```python
from build123d import *

# Parameters (mm, degrees)
SKETCH1_W                        = 144
SKETCH1_H                        = 64
BOSS_EXTRUDE1_DEPTH              = 16
SKETCH3_W                        = 26
SKETCH3_H                        = 64
BOSS_EXTRUDE2_DEPTH              = 36
CHAMFER1_SIZE                    = 16
CUT_EXTRUDE1_REACH               = 146
SKETCH5_R                        = 8
BOSS_EXTRUDE3_DEPTH              = 22
FILLET1_R                        = 3
TAP_DRILL_FOR_M6_HELICOIL2_D     = 6.25
TAP_DRILL_FOR_M6_HELICOIL2_DEPTH = 10
TAP_DRILL_FOR_M6_HELICOIL2_TIP   = 1.877689434


with BuildPart() as part:
    # Sketch1 → Boss-Extrude1 (new body)
    with BuildSketch(Plane(origin=(0, 0, 0), x_dir=(1, 0, 0), z_dir=(0, 1, 0))):
        Rectangle(SKETCH1_W, SKETCH1_H)
    extrude(amount=BOSS_EXTRUDE1_DEPTH)

    # Sketch3 → Boss-Extrude2 (add)
    with BuildSketch(Plane(origin=(0, 16, 0), x_dir=(1, 0, 0), z_dir=(0, 1, 0))):
        with Locations((-59, 0)):
            Rectangle(SKETCH3_W, SKETCH3_H)
    extrude(amount=BOSS_EXTRUDE2_DEPTH)

    # Chamfer1
    chamfer1_edges = [part.edges().sort_by_distance(p)[0] for p in [
        (-72, 52, 0),
    ]]
    chamfer(chamfer1_edges, length=CHAMFER1_SIZE)

    # Sketch2 → Cut-Extrude1 (cut, up to next)
    with BuildSketch(Plane(origin=(72, 0, 0), x_dir=(0, 0, -1), z_dir=(1, 0, 0)), mode=Mode.PRIVATE) as cut_extrude1_sk1:
        Polygon((-16, 0), (-16, 7), (-8, 7), (-8, 16), (8, 16), (8, 7), (16, 7), (16, 0), align=None)
    cut_extrude1_tool1 = extrude(cut_extrude1_sk1.sketch, amount=-CUT_EXTRUDE1_REACH, mode=Mode.PRIVATE) & part.part
    add(cut_extrude1_tool1.solids().sort_by_distance((72, 6.630435, 0))[0], mode=Mode.SUBTRACT)

    # Sketch5 → Boss-Extrude3 (add)
    with BuildSketch(Plane(origin=(72, 0, 0), x_dir=(0, 0, -1), z_dir=(1, 0, 0))):
        with BuildLine():
            Line((-14.413228488, 42.946858611), (-27.401020705, 16))
            Line((-27.401020705, 16), (26.567243493, 16))
            Line((26.567243493, 16), (14.586247124, 42.575818949))
            ThreePointArc((14.586247124, 42.575818949), (0.204698485, 51.998690525), (-14.413228488, 42.946858611))
        make_face()
        with Locations((0, 36)):
            Circle(SKETCH5_R, mode=Mode.SUBTRACT)
    extrude(amount=-BOSS_EXTRUDE3_DEPTH)

    # Fillet1
    fillet1_edges = [part.edges().sort_by_distance(p)[0] for p in [
        (61, 16, -26.567243493),
        (61, 16, 27.401020705),
    ]]
    fillet(fillet1_edges, radius=FILLET1_R)

    # Tap Drill for M6 Helicoil2
    with Locations(Plane(origin=(-36, 0, 22), x_dir=(0, 0, -1), z_dir=(0, -1, 0))):
        with Locations((0, 0), (0, 70), (44, 0), (44, 70)):
            Hole(TAP_DRILL_FOR_M6_HELICOIL2_D / 2, depth=TAP_DRILL_FOR_M6_HELICOIL2_DEPTH)
            with Locations((0, 0, -(TAP_DRILL_FOR_M6_HELICOIL2_DEPTH + TAP_DRILL_FOR_M6_HELICOIL2_TIP / 2))):  # 118° drill point
                Cone(0, TAP_DRILL_FOR_M6_HELICOIL2_D / 2, TAP_DRILL_FOR_M6_HELICOIL2_TIP, mode=Mode.SUBTRACT)


solid = part.part
```
Part model, mm, in its own coordinate system. A direction names the side the tool comes from. Round coordinates to 2 decimals unless told otherwise and drop trailing zeros. Write each loop counter-clockwise with the first axis right and the second up, starting at its lowest first coordinate (ties: lowest second). Pieces come first, ordered by that corner, then holes. Notation, with made-up numbers: (83.5, 8.25) -> (119.5, 8.25) arc R20 ccw to (119.5, 16.25) -> close; hole circle Ø1 at (41.5, 58.5). An arc over 180 degrees is marked (long way). Return JSON: item names as keys, results as strings. Group by question number.
Q1. Probe L1, parallel to X at y = 3.75, z = 22 (3 decimals); L2, parallel to Z at x = 34, y = 5 (3 decimals); L3, parallel to Z at x = 65, y = 14. List the from-to ranges inside material, lowest first. Write a range as [from, to].
Q2. Mould opens along X. For faces 5 (the flat face through (-1, 16, 20)), 6 (the flat face through (-59, 16, 0)) say: pulls with the +X half, pulls with the -X half, needs draft (parallel to the pull), parting line crosses it, or undercut.
Q3. Pin check, flat tips, straight feed: pin 1 (8 mm diameter, centred on x = 63, z = 3.5, fed in from -Y); pin 2 (8 mm diameter, centred on x = 34, z = -22, fed in from +Y); pin 3 (4 mm diameter, centred on x = -2.5, z = 12.5, fed in from -Y). Stop position of each tip, or through.
Q4. Saw through at A-A on x = 41.5. Write the cut outline in (y, z), plus the area to 3 significant figures.
Q5. Saw through at C-C on z = 0. Write the cut outline in (x, y).
Q6. Which spindle directions (+Z, -Z, +X, -X, +Y, -Y) get a long thin tool onto all of the face, cutting with end or side? Do faces 1 (the flat face through (50, 26, 1)), 2 (the cylindrical face through (61.154, 43.932, 1.041)), 3 (the flat face through (1, 3, 16)), 4 (the cylindrical face through (60.85, 16.47, 27.67)). Say none if no direction does.
Q7. Saw through at D-D on x = -63. Write the cut outline in (y, z).
Q8. Saw through at B-B on y = 46. Write the cut outline in (x, z).
Answer:
{
 "1": {"L1": "[-72, -39.125], [-32.875, 30.875], [37.125, 72]", "L2": "[-32, -25.125], [-18.875, -16], [16, 18.875], [25.125, 32]", "L3": "[-32, -8], [8, 32]"},
 "2": {"face 5": "undercut", "face 6": "needs draft"},
 "3": {"pin 1": "y = 16", "pin 2": "y = 16", "pin 3": "y = 7"},
 "4": {"outline": "(0, -32) -> (16, -32) -> (16, -8) -> (7, -8) -> (7, -16) -> (0, -16) -> close; (0, 16) -> (7, 16) -> (7, 8) -> (16, 8) -> (16, 32) -> (0, 32) -> close", "area": "656 mm2"},
 "5": {"outline": "(-72, 16) -> (-46, 16) -> (-46, 52) -> (-56, 52) -> (-72, 36) -> close; (50, 16) -> (72, 16) -> (72, 28) -> (50, 28) -> close; (50, 44) -> (72, 44) -> (72, 52) -> (50, 52) -> close"},
 "6": {"face 1": "+Z, -Z, +Y", "face 2": "+X", "face 3": "+X, -X, -Y", "face 4": "+Z, +X, +Y"},
 "7": {"outline": "(0, -32) -> (45, -32) -> (45, 32) -> (0, 32) -> (0, 16) -> (7, 16) -> (7, 8) -> (16, 8) -> (16, -8) -> (7, -8) -> (7, -16) -> (0, -16) -> close"},
 "8": {"outline": "(-62, -32) -> (-46, -32) -> (-46, 32) -> (-62, 32) -> close; (50, -12.49) -> (72, -12.49) -> (72, 12.49) -> (50, 12.49) -> close"}
}
